Part model, mm, in its own coordinate system. Coordinates: 2 decimals unless noted, no trailing zeros. Order: outer loops, then holes, each group sorted by start corner. A loop starts at its lowest first (then second) coordinate and runs counter-clockwise, first axis right, second up. Notation, with made-up numbers: M 0.5,87.5 L 26.5,87.5 A26 cw 26.5,102.5 Z; hole C 43.25,5 d8. An arc over 180 degrees is marked long. Write item = value, one per line. Start each with the question number.
from build123d import *

# Parameters (mm, degrees)
SKETCH1_R           = 3.2639
BOSS_EXTRUDE1_DEPTH = 3.175
CAVITY1_OUTLINE_W   = 11.43
CAVITY1_OUTLINE_H   = 8.831388176
FILLET3_R           = 1.27


# Read off the part's stored shape, not the designer's step: Cavity1
with BuildPart() as part:
    # Sketch1 → Boss-Extrude1 (new body)
    with BuildSketch(Plane.XY):
        with BuildLine():
            ThreePointArc((9.430957534, 1.335164779), (0, 9.525), (-9.430957534, 1.335164779))
            Line((-9.430957534, 1.335164779), (-14.605, -35.211766))
            Line((-14.605, -35.211766), (14.605, -35.211766))
            Line((14.605, -35.211766), (9.430957534, 1.335164779))
        make_face()
        Circle(SKETCH1_R, mode=Mode.SUBTRACT)
    extrude(amount=BOSS_EXTRUDE1_DEPTH)

    # Cavity1 outline → Cavity1 (revolve, cut)
    with BuildSketch(Plane(origin=(-1.130247142, -31.06550514, 11.268870294), x_dir=(0.995594734936216, 0.03225653994771549, 0.08803771576936452), z_dir=(0, 0.9389588693345029, -0.34402941981474794))):
        with Locations((5.715, 8.721306361)):
            Rectangle(CAVITY1_OUTLINE_W, CAVITY1_OUTLINE_H)
    revolve(axis=Axis((-1.130247142, -31.06550514, 11.268870294), (0.09376099278103864, -0.34251387903072417, -0.9348225066310935)), mode=Mode.SUBTRACT)

    # Fillet3
    fillet3_edges = [part.edges().sort_by_distance(p)[0] for p in [
        (-14.605, -35.211766, 1.5875),
        (14.605, -35.211766, 1.5875),
    ]]
    fillet(fillet3_edges, radius=FILLET3_R)


solid = part.part
Item 1: Cut at B-B, the plane y = -20. Write the cut outline in (x, z) (3 decimals).
Item 2: Flat gauge pins, fed straight in: pin 1 (6 mm diameter, centred on x = 0, y = 0, fed in from +Z); pin 2 (1 mm diameter, centred on y = -24.5, z = 2.5, fed in from -X); pin 3 (1 mm diameter, centred on y = -24.5, z = 1, fed in from +X). Where does each tip first touch, or does it go through?
Item 3: Pull direction X, two halves, no side cores. Call faces 1 (the flat face through (0, -13, 3.175)), 2 (the cylindrical face through (0.191, 9.523, 1.565)), 3 (the cylindrical face through (-0.552, -22.771, 0.683)), 4 (the cylindrical face through (-0.708, -3.186, 1.565)): pulls with the +X half, pulls with the -X half, needs draft (parallel to the pull), parting line crosses it, or undercut.
Item 4: Wall check: line 1 along X through (y, z) = (-1.5, 1.7); line 2 along Y through (x, z) = (-1.75, 1.1); line 3 along X through (y, z) = (-25.5, 1). Give the ranges that are in metal, low to high. Write a range as [from, to].
Item 5: Cut at A-A, the plane y = -1.5. Write the cut outline in (x, z) (3 decimals).
Filled sheet:
q1.outline = M -12.451,0 L 12.451,0 L 12.451,3.175 L -12.451,3.175 Z
q2.pin_1 = through
q2.pin_2 = -13.16
q2.pin_3 = 13.16
q3.face_1 = needs draft
q3.face_2 = parting line crosses it
q3.face_3 = undercut
q3.face_4 = undercut
q4.line_1 = [-9.83, -2.9], [2.9, 9.83]
q4.line_2 = [-22.69, -2.76], [2.76, 9.36]
q4.line_3 = [-13.23, -7.78], [6.97, 13.23]
q5.outline = M -9.832,0 L -2.899,0 L -2.899,3.175 L -9.832,3.175 Z; M 2.899,0 L 9.832,0 L 9.832,3.175 L 2.899,3.175 Z
